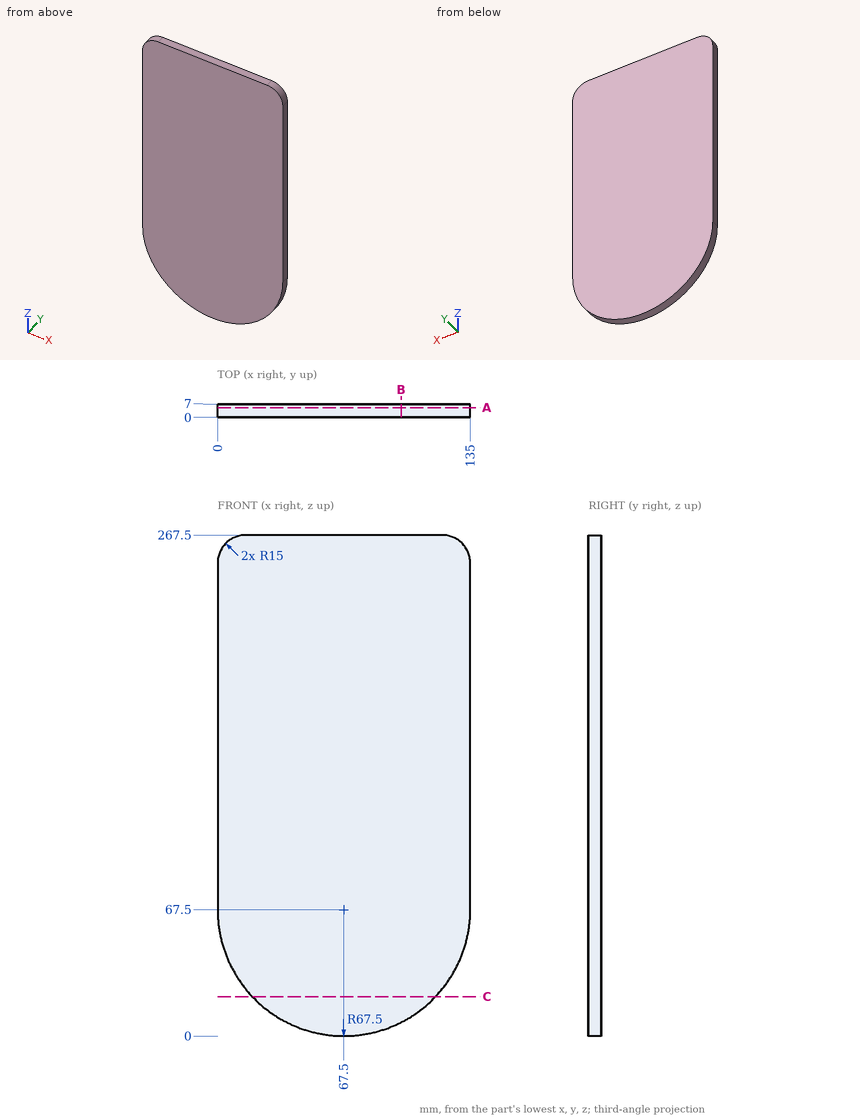
Check sheet for the drawn part. Datum: minimum x, y, z corner. Units: mm. Round coordinates to 2 decimals unless told otherwise and drop trailing zeros. Order: outer loops, then holes, each group sorted by start corner. A loop starts at its lowest first (then second) coordinate and runs counter-clockwise, first axis right, second up. Notation, with made-up numbers: (2, 30) - (46, 30) arc R22 cw to (46, 40) - close; hole circle Ø6 at (2, 47.25). An arc over 180 degrees is marked (long way). Use a Markdown table: item, result. Add a question column.
(1) Sectioned sample at A-A, the plane y = 5. Enter the section's corners in (x, z), and give its area (3 significant figures).
(2) Sectioned sample at C-C, the plane z = 21. Enter the section's corners in (x, y), and give its area (3 significant figures).
(3) Sectioned sample at B-B, the plane x = 98. Enter the section's corners in (y, z), and give its area (3 significant figures).
(4) Depth check by flat-ended pin: pin 1 (1 mm diameter, centred on x = 65, y = 3, fed in from -Z); pin 2 (4 mm diameter, centred on x = 44, y = 5, fed in from -Z). Enter the tip coordinate at first touch or a pass-through.
(5) Material ranges on line 1 along Z through (x, y) = (68, 3.75); line 2 along Z through (x, y) = (98, 3.75); line 3 along X through (y, z) = (5, 256), recorded low to high. Write a range as [from, to].
Answers below:
| question | item | result |
|---|---|---|
| 1 | outline | (0, 67.5) arc R67.5 ccw to (135, 67.5) - (135, 252.5) arc R15 ccw to (120, 267.5) - (15, 267.5) arc R15 ccw to (0, 252.5) - close |
| 1 | area | 34,100 mm² |
| 2 | outline | (18.57, 0) - (116.43, 0) - (116.43, 7) - (18.57, 7) - close |
| 2 | area | 685 mm² |
| 3 | outline | (0, 7.28) - (7, 7.28) - (7, 267.5) - (0, 267.5) - close |
| 3 | area | 1,820 mm² |
| 4 | pin 1 | z = 0.03 |
| 4 | pin 2 | z = 3.52 |
| 5 | line 1 | [0, 267.5] |
| 5 | line 2 | [7.28, 267.5] |
| 5 | line 3 | [0.41, 134.59] |
